from build123d import *

# Parameters (mm, degrees)
F0_R     = 104
F1_DEPTH = 14.9
F2_R     = 80
F3_DEPTH = 14.1
F4_SIZE  = 2
F6_D     = 149
F8_D     = 14


with BuildPart() as f1:
    # F0 (on Right) → F1 (new body)
    with BuildSketch(Plane.YZ):
        Circle(F0_R)
    extrude(amount=F1_DEPTH)

    # F2 (on face) → F3 (join)
    with BuildSketch(Plane(origin=(0, 0, 0), x_dir=(0, -1, 0), z_dir=(-1, 0, 0))):
        Circle(F2_R)
    extrude(amount=F3_DEPTH)

    # F4
    f4_edges = [f1.edges().sort_by_distance(p)[0] for p in [
        (-14.1, 80, 0),
    ]]
    chamfer(f4_edges, length=F4_SIZE)

    # F6 (through all)
    with Locations(Plane.YZ.offset(14.9)):
        with Locations((0, 0)):
            Hole(F6_D / 2)

    # F8 (through all)
    with Locations(Plane.YZ.offset(14.9)):
        with Locations((93, 0), (0, -93), (-93, 0), (0, 93)):
            Hole(F8_D / 2)


solid = f1.part
Build history of the part. All positions in model axes, mm. A direction names the side the tool comes from. Give positions to 0.01 mm unless a question says otherwise; leave off trailing zeros. Loops run counter-clockwise (first coordinate to the right, second up) from the corner with the lowest first, then second, coordinate; pieces in that order, holes last. Notation, with made-up numbers: (2.25, 47.5) - (11.25, 47.5) arc R23 ccw to (11.25, 71.5) - close; hole circle Ø8 at (-13, 32.25). An arc over 180 degrees is marked (long way). Write item = value, one per line. Start each with the question number.
1) Drop flat-ended pins along their axis: pin 1 Ø8 at (x, z) = (0, -81) entering from -Y; pin 2 Ø8 at (x, y) = (-7.5, -11.5) entering from +Z; pin 3 Ø16 at (y, z) = (0, 93) entering from -X; pin 4 Ø12.5 at (y, z) = (-93, 0) entering from +X. Give the stop position or say it passes through.
2) Band-saw the part on A-A on y = 0. Give the cut face in (x, z), plus the area to 3 significant figures.
3) Tool access for faces 4 (the cylindrical face through (0.2, -71.06, 22.38)), 5 (the cylindrical face through (-5.97, 17.34, -78.1)): list every direction of +Z, -Z, +X, -X, +Y, -Y with a clear straight run to the whole face (end or side of a thin tool).
4) Pull direction Z, two halves, no side cores. Call faces 1 (the flat face through (14.9, 30, -69)), 2 (the cylindrical face through (7.346, -82.531, -63.282)), 3 (the cylindrical face through (7.35, 0.91, -86.06)): +Z half, -Z half, draft (parallel to the pull), parting line (faces both ways), or undercut.
5) Band-saw the part on D-D on y = 93. Give the cut face in (x, z), plus the area to 3 significant figures.
6) Probe probe 1 along Z at (x, y) = (6.25, 0); probe 2 along X at (y, z) = (92, -42.5); probe 3 along Y at (x, z) = (3.75, 17). List the from-to ranges inside material, lowest first. Write a range as from..to.
7) Band-saw the part on B-B on x = 3. Give the cut face in (y, z), plus the area to 3 significant figures.
Final values:
q1.pin_1 = -69.91
q1.pin_2 = 79.65
q1.pin_3 = 0
q1.pin_4 = through
q2.outline = (-14.1, -78) - (-12.1, -80) - (0, -80) - (0, -86) - (14.9, -86) - (14.9, -74.5) - (-14.1, -74.5) - close; (-14.1, 74.5) - (14.9, 74.5) - (14.9, 86) - (0, 86) - (0, 80) - (-12.1, 80) - (-14.1, 78) - close; (0, -104) - (14.9, -104) - (14.9, -100) - (0, -100) - close; (0, 100) - (14.9, 100) - (14.9, 104) - (0, 104) - close
q2.area = 613 mm²
q3.face_4 = +X, -X
q3.face_5 = -X
q4.face_1 = draft
q4.face_2 = parting line
q4.face_3 = undercut
q5.outline = (0, -46.55) - (14.9, -46.55) - (14.9, -7) - (0, -7) - close; (0, 7) - (14.9, 7) - (14.9, 46.55) - (0, 46.55) - close
q5.area = 1,180 mm²
q6.probe_1 = -104..-100, -86..-74.5, 74.5..86, 100..104
q6.probe_2 = 0..14.9
q6.probe_3 = -102.6..-72.53, 72.53..102.6
q7.outline = circle Ø208 at (0, 0); hole circle Ø14 at (-93, 0); hole circle Ø149 at (0, 0); hole circle Ø14 at (0, -93); hole circle Ø14 at (0, 93); hole circle Ø14 at (93, 0)
q7.area = 15,900 mm²
